Input: part model. Units: mm. Frame: model coordinates. A direction names the side the tool comes from. Round coordinates to 2 decimals unless told otherwise and drop trailing zeros. Loops run counter-clockwise (first coordinate to the right, second up) from the corner with the lowest first, then second, coordinate; pieces in that order, holes last. Notation, with made-up numbers: (12, 23.5) -> (71, 23.5) arc R10 cw to (71, 42.5) -> close; hole circle Ø2 at (19.5, 76). An arc over 180 degrees is marked (long way). Answer as a JSON object with one key per item and string values. Group by question number.
Item 1: Section query C-C on y = -60. Count the separate pieces of the cut face and the enclosed holes in it, and give its area (3 significant figures).
Item 2: Set-up query: faces 1 (the flat face through (-18, -25, 54)), 2 (the flat face through (195, -67, 20)), 3 (the flat face through (76, -1, 0)). Return all of +Z, -Z, +X, -X, +Y, -Y with unobstructed straight access to the full face (end or side cutting, diameter ignored); none if empty.
Item 3: Section query D-D on z = 30. Return loops of the section in (x, y).
Item 4: Pin query (flat end, axial travel): pin 1 (25 mm diameter, centred on x = 68, y = 60, fed in from +Z); pin 2 (25 mm diameter, centred on x = 181.5, y = -54, fed in from +Z); pin 3 (19.5 mm diameter, centred on y = 72, z = 200, fed in from +X). Return the tip coordinate at first contact, or that it passes through.
Item 5: Section query A-A on z = 128. Return loops of the section in (x, y).
Item 6: Section query B-B on y = 60. Return loops of the section in (x, z).
Item 7: Material intervals for line 1 (X direction, y = 65, z = 251.5); line 2 (Z direction, x = 67, y = 45); line 3 (Y direction, x = -12, z = 41), sorted ascending. Write a range as [from, to].
Item 8: Draft query along Y for faces 4 (the cylindrical face through (-55.02, -56.45, 248.86)), 5 (the flat face through (-32.23, -1, 145)), 6 (the cylindrical face through (-52.51, 69.929, 271.484)), 7 (the flat face through (195, 53, 20)). Return one class per face: released by +Y, released by -Y, zero draft, split by the parting line, or undercut.
from build123d import *

# Parameters (mm, degrees)
F1_DEPTH  = 100
F2_R      = 99.99999
F3_R      = 8.75
F4_DEPTH  = 40.001
F3_R_2    = 15.75
F5_DEPTH  = 20
F6_R      = 50
F7_DEPTH  = 40.001
F11_DEPTH = 25
F12_R     = 10
F13_D     = 12.1
F16_D     = 12.1
F16_DEPTH = 69.85
F16_START = 0.1831763
F16_TIP   = 3.6352067451


# Not quite as in the source:
# - a fillet or chamfer is up to 0.001 mm smaller than in the source, because OpenCascade refuses the exact size


with BuildPart() as f1:
    # F0 (on Front) → F1 (new body, symmetric)
    with BuildSketch(Plane.XZ):
        Polygon((-72.2300410013, 0), (227.7699589987, 0), (227.7699589987, 40), (-32.2300410013, 40), (-32.2300410013, 300), (-72.2300410013, 300), align=None)
    extrude(amount=F1_DEPTH, both=True)

    # F2 (radius 100 in the source; OpenCascade refuses exactly that, so slightly less here)
    f2_edges = [f1.edges().sort_by_distance(p)[0] for p in [
        (-52.230041, -100, 300),
        (-52.230041, 100, 300),
    ]]
    fillet(f2_edges, radius=F2_R)

    # F3 (on face) → F4 (cut, through all)
    with BuildSketch(Plane.XY.offset(40)):
        with Locations((67.7699589987, 60)):
            Circle(F3_R)
        with Locations((187.7699589987, 60)):
            Circle(F3_R)
        with Locations((67.7699589987, -60)):
            Circle(F3_R)
        with Locations((187.7699589987, -60)):
            Circle(F3_R)
    extrude(amount=-F4_DEPTH, mode=Mode.SUBTRACT)

    # F3 (on face) → F5 (cut)
    with BuildSketch(Plane.XY.offset(40)):
        with Locations((187.7699589987, 60)):
            Circle(F3_R_2)
        with Locations((187.7699589987, 60)):
            Circle(F3_R, mode=Mode.SUBTRACT)
        with Locations((67.7699589987, 60)):
            Circle(F3_R_2)
        with Locations((67.7699589987, 60)):
            Circle(F3_R, mode=Mode.SUBTRACT)
        with Locations((67.7699589987, -60)):
            Circle(F3_R_2)
        with Locations((67.7699589987, -60)):
            Circle(F3_R, mode=Mode.SUBTRACT)
        with Locations((187.7699589987, -60)):
            Circle(F3_R_2)
        with Locations((187.7699589987, -60)):
            Circle(F3_R, mode=Mode.SUBTRACT)
    extrude(amount=-F5_DEPTH, mode=Mode.SUBTRACT)

    # F6 (on face) → F7 (cut, through all)
    with BuildSketch(Plane.YZ.offset(-32.2300410013)):
        with Locations((0, 200)):
            Circle(F6_R)
    extrude(amount=-F7_DEPTH, mode=Mode.SUBTRACT)

    # F10 (on offset) → F11 (join, symmetric)
    with BuildSketch(Plane(origin=(0, 0, 0), x_dir=(-1, 0, 0), z_dir=(0, 1, 0))):
        Polygon((-17.1466749161, 40), (32.2300410013, 40), (32.2300410013, 89.3767159174), align=None)
    extrude(amount=F11_DEPTH, both=True)

    # F12
    f12_edges = [f1.edges().sort_by_distance(p)[0] for p in [
        (-32.230041, 62.5, 40),
        (-32.230041, -62.5, 40),
    ]]
    fillet(f12_edges, radius=F12_R)

    # F13 (through all)
    with Locations(Plane.YZ.offset(-32.2300410013)):
        with Locations((0, 272), (72, 200), (0, 128), (-72, 200)):
            Hole(F13_D / 2)

    # F16
    # its depths count from where the whole tool has entered the part; down to there all is cleared
    with Locations(Plane(origin=(0, -170.7106781187, 170.7106781187), x_dir=(1, 0, 0), z_dir=(0, -0.7071067812, 0.7071067812)).offset(-F16_START)):
        with Locations((-52.2300410013, 141.4213562373)):
            Hole(F16_D / 2, depth=F16_DEPTH)
            with Locations((0, 0, -(F16_DEPTH + F16_TIP / 2))):  # 118° drill point
                Cone(0, F16_D / 2, F16_TIP, mode=Mode.SUBTRACT)


solid = f1.part
Solved:
{
 "1": {"separate pieces": "3", "enclosed holes": "1", "area": "19,500 mm²"},
 "2": {"face 1": "+Z, +X, -Y", "face 2": "+Z", "face 3": "-Z, +X, -X, +Y, -Y"},
 "3": {"outline": "(-72.23, -100) -> (227.77, -100) -> (227.77, 100) -> (-72.23, 100) -> close; hole circle Ø31.5 at (67.77, -60); hole circle Ø31.5 at (67.77, 60); hole circle Ø31.5 at (187.77, -60); hole circle Ø31.5 at (187.77, 60)"},
 "4": {"pin 1": "z = 20", "pin 2": "z = 40", "pin 3": "x = -32.23"},
 "5": {"outline": "(-72.23, -100) -> (-32.23, -100) -> (-32.23, -6.05) -> (-72.23, -6.05) -> close; (-72.23, 6.05) -> (-32.23, 6.05) -> (-32.23, 100) -> (-72.23, 100) -> close"},
 "6": {"outline": "(-72.23, 0) -> (59.02, 0) -> (59.02, 20) -> (52.02, 20) -> (52.02, 40) -> (-22.23, 40) arc R10 cw to (-32.23, 50) -> (-32.23, 280) -> (-72.23, 280) -> close; (76.52, 0) -> (179.02, 0) -> (179.02, 20) -> (172.02, 20) -> (172.02, 40) -> (83.52, 40) -> (83.52, 20) -> (76.52, 20) -> close; (196.52, 0) -> (227.77, 0) -> (227.77, 40) -> (203.52, 40) -> (203.52, 20) -> (196.52, 20) -> close"},
 "7": {"line 1": "[-72.23, -32.23]", "line 2": "[0, 20]", "line 3": "[-25, 25]"},
 "8": {"face 4": "undercut", "face 5": "zero draft", "face 6": "released by +Y", "face 7": "undercut"}
}
